```python
from build123d import *

# Parameters (mm, degrees)
F0_W     = 74
F0_H     = 85
F0_R     = 3
F0_R_2   = 4
F1_DEPTH = 12
F2_R     = 7
F3_DEPTH = 6
F4_W     = 2
F4_H     = 6
F5_DEPTH = 2
F6_R     = 9
F7_DEPTH = 5
F8_R     = 4
F9_DEPTH = 0.5
F10_R    = 5
F11_R    = 2


with BuildPart() as f1:
    # F0 (on Front) → F1 (new body)
    with BuildSketch(Plane.XZ):
        Rectangle(F0_W, F0_H)
        with Locations((-19.7989898732, -24.7989898732)):
            Circle(F0_R, mode=Mode.SUBTRACT)
        Polygon((-17.7320508076, -1), (-16, 2), (-14.2679491924, -1), align=None, mode=Mode.SUBTRACT)
        Circle(F0_R_2, mode=Mode.SUBTRACT)
        Polygon((14.2679491924, -1), (16, 2), (17.7320508076, -1), align=None, mode=Mode.SUBTRACT)
        with Locations((19.7989898732, 14.7989898732)):
            Circle(F0_R, mode=Mode.SUBTRACT)
    extrude(amount=F1_DEPTH)

    # F2 (on face) → F3 (cut)
    with BuildSketch(Plane.XZ.offset(12)):
        with Locations((19.7989898732, 14.7989898732)):
            Circle(F2_R)
        with Locations((-19.7989898732, -24.7989898732)):
            Circle(F2_R)
    extrude(amount=-F3_DEPTH, mode=Mode.SUBTRACT)

    # F4 (on Right) → F5 (cut, symmetric)
    with BuildSketch(Plane.YZ):
        with Locations((-1, -39.5)):
            Rectangle(F4_W, F4_H)
    extrude(amount=F5_DEPTH, both=True, mode=Mode.SUBTRACT)

    # F6 (on face) → F7 (cut)
    with BuildSketch(Plane(origin=(0, 0, 0), x_dir=(-1, 0, 0), z_dir=(0, 1, 0))):
        Circle(F6_R)
    extrude(amount=-F7_DEPTH, mode=Mode.SUBTRACT)

    # F8 (on face) → F9 (join)
    with BuildSketch(Plane(origin=(0, -5, 0), x_dir=(-1, 0, 0), z_dir=(0, 1, 0))):
        Circle(F8_R)
    extrude(amount=-F9_DEPTH)

    # F10
    f10_edges = [f1.edges().sort_by_distance(p)[0] for p in [
        (0, -12, 42.5),
        (-37, -12, 0),
        (37, -12, 0),
        (0, -12, -42.5),
        (37, -6, -42.5),
        (37, -6, 42.5),
        (-37, -6, 42.5),
        (-37, -6, -42.5),
    ]]
    fillet(f10_edges, radius=F10_R)

    # F11
    f11_edges = [f1.edges().sort_by_distance(p)[0] for p in [
        (9, 0, 0),
        (-4, -12, 0),
    ]]
    fillet(f11_edges, radius=F11_R)


solid = f1.part
```
Read the model definition and answer for the solid it produces. Units are mm, in the model's axes. A direction names the side the tool comes from. Round coordinates to 2 decimals unless told otherwise and drop trailing zeros. Loops run counter-clockwise (first coordinate to the right, second up) from the corner with the lowest first, then second, coordinate; pieces in that order, holes last. Notation, with made-up numbers: (85, 15.25) -> (130, 15.25) arc R27 ccw to (130, 38.25) -> close; hole circle Ø2 at (-23, -27.5). An arc over 180 degrees is marked (long way). One line per item, written item: value.
1) Consider L1, parallel to X at y = -6.75, z = 0; L2, parallel to Z at x = -16.5, y = -10; L3, parallel to Z at x = 0, y = -6.6. Determine where each line is inside the solid, lowest interval first. Write a range as [from, to].
Answer list:
L1: x = [-37, -17.15], [-14.85, -4], [4, 14.85], [17.15, 37]
L2: z = [-41.5, -30.97], [-18.63, -1], [1.13, 41.5]
L3: z = [-42.5, -4], [4, 42.5]
2) A cutting plane is placed at A-A (z = 0). Determine the outline of the cut face in (x, y), and give its area (3 significant figures).
Answer list:
outline: (-37, -7) arc R5 ccw to (-32, -12) -> (-17.15, -12) -> (-17.15, 0) -> (-37, 0) -> close; (-14.85, -12) -> (-6, -12) arc R2 ccw to (-4, -10) -> (-4, -5.5) -> (4, -5.5) -> (4, -10) arc R2 ccw to (6, -12) -> (14.85, -12) -> (14.85, 0) -> (11, 0) arc R2 ccw to (9, -2) -> (9, -5) -> (-9, -5) -> (-9, -2) arc R2 ccw to (-11, 0) -> (-14.85, 0) -> close; (17.15, -12) -> (32, -12) arc R5 ccw to (37, -7) -> (37, 0) -> (17.15, 0) -> close
area: 676 mm²
3) Flat-ended cylindrical pins translate along their axes: P1, Ø2, axis at y = -1.5, z = -40.5, coming from the +X side; P2, Ø1.6, axis at x = 0.5, y = -0.5, coming from the -Z side; P3, Ø14.5, axis at x = -2, z = -2.5, coming from the +Y side; P4, Ø5, axis at x = 19.8, z = 14.8, coming from the +Y side. Find the tip coordinate at first contact, or state that the pin passes through.
Answer list:
P1: stops at x = 36.58
P2: stops at z = -36.5
P3: stops at y = -0.08
P4: passes through
4) A cutting plane is placed at B-B (x = -21.5). Determine the outline of the cut face in (y, z), and give its area (3 significant figures).
Answer list:
outline: (-12, -37.5) arc R5 ccw to (-7, -42.5) -> (0, -42.5) -> (0, -27.27) -> (-6, -27.27) -> (-6, -31.59) -> (-12, -31.59) -> close; (-12, -18.01) -> (-6, -18.01) -> (-6, -22.33) -> (0, -22.33) -> (0, 42.5) -> (-7, 42.5) arc R5 ccw to (-12, 37.5) -> close
area: 898 mm²
5) A cutting plane is placed at C-C (x = 0). Determine the outline of the cut face in (y, z).
Answer list:
outline: (-12, -37.5) arc R5 ccw to (-7, -42.5) -> (-2, -42.5) -> (-2, -36.5) -> (0, -36.5) -> (0, -11) arc R2 ccw to (-2, -9) -> (-5, -9) -> (-5, 9) -> (-2, 9) arc R2 ccw to (0, 11) -> (0, 42.5) -> (-7, 42.5) arc R5 ccw to (-12, 37.5) -> (-12, 6) arc R2 ccw to (-10, 4) -> (-5.5, 4) -> (-5.5, -4) -> (-10, -4) arc R2 ccw to (-12, -6) -> close
6) The mould has two halves that part along Z. Classify faces 4 (the face through (0, -3, 42.5)), 5 (the face through (1.172, -3.479, 8.923)), 6 (the face through (-35.5, -3.55, -41.07)): pulls with the +Z half, pulls with the -Z half, needs draft (parallel to the pull), parting line crosses it, or undercut.
Answer list:
face 4: pulls with the +Z half
face 5: undercut
face 6: pulls with the -Z half
7) For faces 1 (the face through (0, -5, 0)), 2 (the face through (23, -6, 15)), 3 (the face through (35.57, -3.55, -41)), determine the directions among +Z, -Z, +X, -X, +Y, -Y from which every point of the face is accessible in a straight line to the end or side of a thin tool.
Answer list:
face 1: +Y
face 2: -Y
face 3: -Z, +X, +Y, -Y
8) A cutting plane is placed at D-D (y = -11). Determine the outline of the cut face in (x, z), and give its area (3 significant figures).
Answer list:
outline: (-35, -37.5) arc R3 ccw to (-32, -40.5) -> (32, -40.5) arc R3 ccw to (35, -37.5) -> (35, 37.5) arc R3 ccw to (32, 40.5) -> (-32, 40.5) arc R3 ccw to (-35, 37.5) -> close; hole circle Ø14 at (-19.8, -24.8); hole (-17.73, -1) -> (-14.27, -1) -> (-16, 2) -> close; hole circle Ø8.54 at (0, 0); hole circle Ø14 at (19.8, 14.8); hole (14.27, -1) -> (17.73, -1) -> (16, 2) -> close
area: 5,290 mm²
